Build history of the part. All positions in model axes, mm. Face numbers are marked on the shaded views. A direction names the side the tool comes from. Coordinates: 2 decimals unless noted, no trailing zeros. Write each loop counter-clockwise with the first axis right and the second up, starting at its lowest first coordinate (ties: lowest second). Pieces come first, ordered by that corner, then holes. Notation, with made-up numbers: (35.5, 64.5) -> (46.5, 64.5) arc R15 ccw to (46.5, 82.5) -> close; hole circle Ø5 at (38.5, 13). An arc over 180 degrees is marked (long way). Write each question's results on one line, items separated by ' | '. Start each with the question number.
Q1. Saw through at B-B on z = 31. Give the cut face in (x, y).
Q2. Saw through at A-A on y = -4.25. Give the cut face in (x, z).
Q3. Tool access for the marked faces 1, 2, 3, 4 and 5: list every direction of +Z, -Z, +X, -X, +Y, -Y with a clear straight run to the whole face (end or side of a thin tool).
Q4. Two-plate mould, pull along X, no slides. Class the marked faces 6, 7, 8 and 9: released by +X, released by -X, zero draft, split by the parting line, or undercut.
Q5. Drill centre lines: line 1 (Y direction, x = 0, z = 8); line 2 (Y direction, x = -47, z = 11); line 3 (Z direction, x = -2, y = -3.5). Where is each one in solid material? Low to high.
Q6. Drop flat-ended pins along their axis: pin 1 Ø10 at (y, z) = (-7, 30) entering from +X; pin 2 Ø3 at (x, y) = (-7.5, -6) entering from -Z; pin 3 Ø4 at (x, y) = (-7.5, -3.5) entering from +Z; pin 4 Ø17.5 at (x, z) = (-44.5, 37.79) entering from -Y. Give the stop position or say it passes through.
Q7. Saw through at D-D on x = -2.5. Give the cut face in (y, z).
Q8. Saw through at C-C on y = -20.25. Give the cut face in (x, z), and give its area (3 significant figures).
from build123d import *

# Parameters (mm, degrees)
F1_DEPTH  = 25.4
F3_DEPTH  = 25.4
F5_DEPTH  = 12.7
F6_R      = 7.5359717886
F7_DEPTH  = 25.4
F9_DEPTH  = 25.4
F11_DEPTH = 13.208
F12_R     = 3.5651940515
F12_R_2   = 3.719082418
F13_DEPTH = 25.4
F14_R     = 3.972943494
F15_DEPTH = 25.4


# Not quite as in the source:
# - a feature names something its author has since deleted; it is built from what else it names


with BuildPart() as f1:
    # F0 (on Front) → F1 (new body)
    with BuildSketch(Plane.XZ):
        Polygon((-56.0294090864, 50.8), (-56.0294090864, 0), (7.4705909136, 0), (7.4705909136, 12.7), (-30.6294090864, 12.7), (-30.6294090864, 50.8), align=None)
    extrude(amount=F1_DEPTH)

    # F2 (on face) → F3 (cut)
    with BuildSketch(Plane.XZ.offset(25.4)):
        with BuildLine():
            ThreePointArc((-56.0294090864, 44.6911064088), (-53.33876103, 48.8568702153), (-48.7761497498, 50.8))
            Line((-48.7761497498, 50.8), (-56.0294090864, 50.8))
            Line((-56.0294090864, 50.8), (-56.0294090864, 44.6911064088))
        make_face()
        with BuildLine():
            Line((-30.6294090864, 50.8), (-37.9370041192, 50.8))
            ThreePointArc((-37.9370041192, 50.8), (-32.7129588614, 47.2060747706), (-30.6294090864, 41.2172712386))
            Line((-30.6294090864, 41.2172712386), (-30.6294090864, 50.8))
        make_face()
    extrude(amount=-F3_DEPTH, mode=Mode.SUBTRACT)

    # F4 (on face) → F5 (cut)
    with BuildSketch(Plane.XZ.offset(25.4)):
        with BuildLine():
            Line((-56.0294090864, 12.7), (-30.6294090864, 12.7))
            Line((-30.6294090864, 12.7), (-30.6294090864, 41.2172712386))
            ThreePointArc((-30.6294090864, 41.2172712386), (-32.7129588614, 47.2060747706), (-37.9370041192, 50.8))
            Line((-37.9370041192, 50.8), (-48.7761497498, 50.8))
            ThreePointArc((-48.7761497498, 50.8), (-53.33876103, 48.8568702153), (-56.0294090864, 44.6911064088))
            Line((-56.0294090864, 44.6911064088), (-56.0294090864, 12.7))
        make_face()
    extrude(amount=-F5_DEPTH, mode=Mode.SUBTRACT)

    # F6 (on face) → F7 (cut)
    with BuildSketch(Plane.XZ.offset(12.7)):
        with Locations((-44.4975420833, 37.7943851054)):
            Circle(F6_R)
    extrude(amount=-F7_DEPTH, mode=Mode.SUBTRACT)

    # F8 (on face) → F9 (cut)
    with BuildSketch(Plane.XY.offset(12.7)):
        with BuildLine():
            Line((-56.0294090864, -25.4), (-50.4875965416, -25.4))
            ThreePointArc((-50.4875965416, -25.4), (-54.4030732732, -23.3868988254), (-56.0294090864, -19.2956195392))
            Line((-56.0294090864, -19.2956195392), (-56.0294090864, -25.4))
        make_face()
        with BuildLine():
            ThreePointArc((7.4705909136, -18.6832621694), (4.6896834238, -23.1031347869), (0, -25.4))
            Line((0, -25.4), (7.4705909136, -25.4))
            Line((7.4705909136, -25.4), (7.4705909136, -18.6832621694))
        make_face()
    extrude(amount=-F9_DEPTH, mode=Mode.SUBTRACT)

    # F10 (on face) → F11 (join)
    with BuildSketch(Plane(origin=(0, 0, 0), x_dir=(-1, 0, 0), z_dir=(0, 1, 0))):
        with BuildLine():
            ThreePointArc((30.6294090864, 22.9618716985), (27.6481288956, 16.3576173964), (21.3930476457, 12.7))
            Line((21.3930476457, 12.7), (30.6294090864, 12.7))
            Line((30.6294090864, 12.7), (30.6294090864, 22.9618716985))
        make_face()
    extrude(amount=-F11_DEPTH)

    # F12 (on face) → F13 (cut)
    with BuildSketch(Plane.XY.offset(12.7)):
        with Locations((-47.0647066832, -18.9685039222)):
            Circle(F12_R)
        with Locations((0, -18.6832621694)):
            Circle(F12_R_2)
    extrude(amount=-F13_DEPTH, mode=Mode.SUBTRACT)

    # F14 (on face) → F15 (cut)
    with BuildSketch(Plane.XY.offset(12.7)):
        with Locations((0, -6.9883959368)):
            Circle(F14_R)
    extrude(amount=-F15_DEPTH, mode=Mode.SUBTRACT)


solid = f1.part
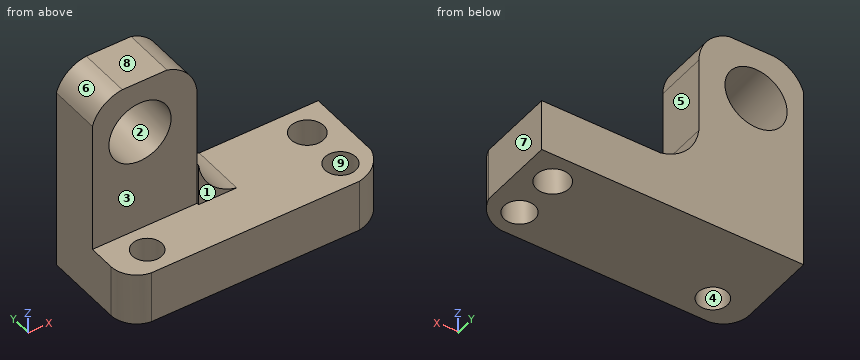
Returned:
1) outline: (-56.03, -12.7) -> (-47.76, -12.7) -> (-47.76, 0) -> (-56.03, 0) -> close; (-41.24, -12.7) -> (-30.63, -12.7) -> (-30.63, 0) -> (-41.24, 0) -> close
2) outline: (-56.03, 0) -> (-2.88, 0) -> (-2.88, 12.7) -> (-21.39, 12.7) arc R11.92 cw to (-30.63, 22.96) -> (-30.63, 41.22) arc R10.18 ccw to (-37.94, 50.8) -> (-48.78, 50.8) arc R8.46 ccw to (-56.03, 44.69) -> close; (2.88, 0) -> (7.47, 0) -> (7.47, 12.7) -> (2.88, 12.7) -> close; hole circle Ø15.07 at (-44.5, 37.79)
3) face 1: +Z, +X, -X, -Y | face 2: +Y, -Y | face 3: +Z, -X, -Y | face 4: +Z, -Z | face 5: +Z, +X, +Y, -Y
4) face 6: released by -X | face 7: released by +X | face 8: zero draft | face 9: undercut
5) line 1: y = -25.4 to -22.4, -14.96 to -10.96, -3.02 to 0 | line 2: y = -25.4 to -22.53, -15.4 to 0 | line 3: z = 0 to 12.7
6) pin 1: stops at x = -30.63 | pin 2: stops at z = 0 | pin 3: stops at z = 12.7 | pin 4: stops at y = -12.7
7) outline: (-25.4, 0) -> (-21.44, 0) -> (-21.44, 12.7) -> (-25.4, 12.7) -> close; (-15.93, 0) -> (-10.08, 0) -> (-10.08, 12.7) -> (-15.93, 12.7) -> close; (-3.9, 0) -> (0, 0) -> (0, 12.7) -> (-3.9, 12.7) -> close
8) outline: (-55.94, 0) -> (-50.39, 0) -> (-50.39, 12.7) -> (-55.94, 12.7) -> close; (-43.74, 0) -> (-3.37, 0) -> (-3.37, 12.7) -> (-43.74, 12.7) -> close; (3.37, 0) -> (6.86, 0) -> (6.86, 12.7) -> (3.37, 12.7) -> close | area: 627 mm2
